```python
from build123d import *

# Parameters (mm, degrees)
F1_DEPTH = 1


with BuildPart() as f1:
    # F0 (on Top) → F1 (new body)
    with BuildSketch(Plane.XY):
        Polygon((-25.5, -5.75), (-25.5, 5.75), (-26.50612, 5.75), align=None)
        Polygon((25.5, 5.75), (-25.5, 5.75), (-25.5, -5.75), (-9.25, -5.75), (-9.25, 2.25), (-7.75, 2.25), (-7.75, -4.25), (7.75, -4.25), (7.75, 2.25), (9.25, 2.25), (9.25, -5.75), (25.5, -5.75), align=None)
        Polygon((26.50612, 5.75), (25.5, 5.75), (25.5, -5.75), align=None)
    extrude(amount=F1_DEPTH)


solid = f1.part
```
The listing builds one solid part. Answer for the finished solid, in the listing's coordinates (mm). A direction names the side the tool comes from. Give positions to 0.01 mm unless a question says otherwise; leave off trailing zeros. Order: outer loops, then holes, each group sorted by start corner. A loop starts at its lowest first (then second) coordinate and runs counter-clockwise, first axis right, second up. Notation, with made-up numbers: (48.5, 72) -> (86.5, 72) arc R17 cw to (86.5, 97) -> close; hole circle Ø2 at (27.5, -40). An arc over 180 degrees is marked (long way). Answer as CSV lines item,"result". Start each with the question number.
Q1. A cutting plane is placed at D-D (y = -1.5). Determine the outline of the cut face in (x, z), then the cut area to 3 significant figures.
Q2. A cutting plane is placed at B-B (z = 0.45). Determine the outline of the cut face in (x, y), then the cut area to 3 significant figures.
Q3. Given pin 1 (0.5 mm diameter, centred on x = -8.5, z = 0.5, fed in from -Y), flat-ended and moving along its own axis, determine where the tip first touches the part or whether it passes through.
Q4. A cutting plane is placed at C-C (x = -2). Determine the outline of the cut face in (y, z).
Q5. Find the intervals of material crossed by L1, parallel to X at y = 1, z = 0.4; L2, parallel to X at y = -1.75, z = 0.5; L3, parallel to Y at x = -6, z = 0.05, in increasing order.
Q6. Determine the mould class of faces 3 (the flat face through (-8.5, 2.25, 0.5)), 4 (the flat face through (0, 0, 0)), 5 (the flat face through (25.996, -0.08, 0.493)) for opening direction X: pulls with the +X half, pulls with the -X half, needs draft (parallel to the pull), parting line crosses it, or undercut.
Q7. A cutting plane is placed at A-A (y = -3.75). Determine the outline of the cut face in (x, z), then the cut area to 4 significant figures.
Q8. Which of the six approach directions +Z, -Z, +X, -X, +Y, -Y give full straight-line access (tool end or side, diameter ignored) to faces 1 (the flat face through (8.5, 2.25, 0.5)), 2 (the flat face through (-26.01, 0.08, 0.49))?
Results found:
1,outline,"(-25.87, 0) -> (-9.25, 0) -> (-9.25, 1) -> (-25.87, 1) -> close; (-7.75, 0) -> (7.75, 0) -> (7.75, 1) -> (-7.75, 1) -> close; (9.25, 0) -> (25.87, 0) -> (25.87, 1) -> (9.25, 1) -> close"
1,area,"48.7 mm2"
2,outline,"(-26.51, 5.75) -> (-25.5, -5.75) -> (-9.25, -5.75) -> (-9.25, 2.25) -> (-7.75, 2.25) -> (-7.75, -4.25) -> (7.75, -4.25) -> (7.75, 2.25) -> (9.25, 2.25) -> (9.25, -5.75) -> (25.5, -5.75) -> (26.51, 5.75) -> close"
2,area,"551 mm2"
3,pin 1,"y = 2.25"
4,outline,"(-4.25, 0) -> (5.75, 0) -> (5.75, 1) -> (-4.25, 1) -> close"
5,L1,"-26.09 to -9.25, -7.75 to 7.75, 9.25 to 26.09"
5,L2,"-25.85 to -9.25, -7.75 to 7.75, 9.25 to 25.85"
5,L3,"-4.25 to 5.75"
6,face 3,"undercut"
6,face 4,"needs draft"
6,face 5,"pulls with the +X half"
7,outline,"(-25.67, 0) -> (-9.25, 0) -> (-9.25, 1) -> (-25.67, 1) -> close; (-7.75, 0) -> (7.75, 0) -> (7.75, 1) -> (-7.75, 1) -> close; (9.25, 0) -> (25.67, 0) -> (25.67, 1) -> (9.25, 1) -> close"
7,area,"48.35 mm2"
8,face 1,"+Z, -Z, -Y"
8,face 2,"+Z, -Z, -X, -Y"
